```python
from build123d import *

# Parameters (mm, degrees)
F1_DEPTH = 45
F2_R     = 7
F3_R     = 4
F4_DEPTH = 3.001
F5_R     = 4
F6_DEPTH = 3.001


with BuildPart() as f1:
    # F0 (on Top) → F1 (new body, symmetric)
    with BuildSketch(Plane.XY):
        Polygon((0, -40), (0, 0), (-40, 0), (-40, -3), (-3, -3), (-3, -40), align=None)
    extrude(amount=F1_DEPTH, both=True)

    # F2
    f2_edges = [f1.edges().sort_by_distance(p)[0] for p in [
        (-3, -3, 0),
        (0, 0, 0),
    ]]
    fillet(f2_edges, radius=F2_R)

    # F3 (on face) → F4 (cut, through all)
    with BuildSketch(Plane.XZ.offset(3)):
        with Locations((-32, 37)):
            Circle(F3_R)
        with Locations((-20, 0)):
            Circle(F3_R)
        with Locations((-32, -37)):
            Circle(F3_R)
    extrude(amount=-F4_DEPTH, mode=Mode.SUBTRACT)

    # F5 (on face) → F6 (cut, through all)
    with BuildSketch(Plane(origin=(-3, 0, 0), x_dir=(0, -1, 0), z_dir=(-1, 0, 0))):
        with Locations((32, 37)):
            Circle(F5_R)
        with Locations((20, 0)):
            Circle(F5_R)
        with Locations((32, -37)):
            Circle(F5_R)
    extrude(amount=-F6_DEPTH, mode=Mode.SUBTRACT)


solid = f1.part
```
Read the model definition and answer for the solid it produces. Units are mm, in the model's axes. A direction names the side the tool comes from. Coordinates: 2 decimals unless noted, no trailing zeros. Loops run counter-clockwise (first coordinate to the right, second up) from the corner with the lowest first, then second, coordinate; pieces in that order, holes last. Notation, with made-up numbers: (28, 52.5) - (81, 52.5) arc R27 cw to (81, 88.5) - close; hole circle Ø6 at (88, -38). An arc over 180 degrees is marked (long way). Answer in a Markdown table with one row per item.
1. Which of the six approach directions +Z, -Z, +X, -X, +Y, -Y give full straight-line access (tool end or side, diameter ignored) to faces 1 (the face through (-25, -3, 1)), 2 (the face through (-23.2, -1.5, -2.4))?
Conclusion:
| item | result |
|---|---|
| face 1 | +Z, -Z, -X, -Y |
| face 2 | +Y, -Y |
2. Given pin 1 (12 mm diameter, centred on x = -19.5, z = 23.5, fed in from -Y); pin 2 (15 mm diameter, centred on y = -22, z = 18.5, fed in from -X); pin 3 (5 mm diameter, centred on y = -32, z = -37, fed in from +X), each flat-ended and moving along its own axis, determine where each tip first touches the part or whether it passes through.
Conclusion:
| item | result |
|---|---|
| pin 1 | stops at y = -3 |
| pin 2 | stops at x = -3 |
| pin 3 | passes through |
3. Find section B-B, the plane z = 37. Write down the section's boundary in (x, y), then the cut area to 3 significant figures.
Conclusion:
| item | result |
|---|---|
| outline | (-40, -3) - (-36, -3) - (-36, 0) - (-40, 0) - close; (-28, -3) - (-10, -3) arc R7 cw to (-3, -10) - (-3, -28) - (0, -28) - (0, -7) arc R7 ccw to (-7, 0) - (-28, 0) - close; (-3, -40) - (0, -40) - (0, -36) - (-3, -36) - close |
| area | 183 mm² |
4. Find section A-A, the plane y = -32. Write down the section's boundary in (x, z), then the cut area to 3 significant figures.
Conclusion:
| item | result |
|---|---|
| outline | (-3, -45) - (0, -45) - (0, -41) - (-3, -41) - close; (-3, -33) - (0, -33) - (0, 33) - (-3, 33) - close; (-3, 41) - (0, 41) - (0, 45) - (-3, 45) - close |
| area | 222 mm² |
5. Straight lines are drawn through the part: line 1 (Z direction, x = -0.65, y = -32); line 2 (Z direction, x = -1, y = -20); line 3 (Y direction, x = -25.5, z = 15). For each, find the intervals that lie inside material, in ascending order.
Conclusion:
| item | result |
|---|---|
| line 1 | z = -45 to -41, -33 to 33, 41 to 45 |
| line 2 | z = -45 to -4, 4 to 45 |
| line 3 | y = -3 to 0 |
6. Find section D-D, the plane y = -20. Write down the section's boundary in (x, z), then the cut area to 3 significant figures.
Conclusion:
| item | result |
|---|---|
| outline | (-3, -45) - (0, -45) - (0, -4) - (-3, -4) - close; (-3, 4) - (0, 4) - (0, 45) - (-3, 45) - close |
| area | 246 mm² |
7. Determine the mould class of faces 3 (the face through (-1.5, -16.8, -2.4)), 4 (the face through (-32.521, -1.521, 40.966)), 5 (the face through (-40, -1, 1)) for opening direction X: +X half, -X half, draft (parallel to the pull), parting line (faces both ways), or undercut.
Conclusion:
| item | result |
|---|---|
| face 3 | draft |
| face 4 | undercut |
| face 5 | -X half |
